```python
from build123d import *

# Parameters (mm, degrees)
BASE_DEPTH                = 12
CASE_MOUNTING_HOLES_REACH = 24.858
SKETCH2_R                 = 1.4
F_1MM_EDGE_FILLETS_R      = 1


with BuildPart() as part:
    # Sketch1 → Base (new body)
    with BuildSketch(Plane(origin=(0, 0, 0), x_dir=(1, 0, 0), z_dir=(0, 1, 0))):
        with BuildLine():
            Line((8.5, 17.5), (8.5, 15.5))
            ThreePointArc((8.5, 15.5), (7.297918472, 15.002081528), (6.8, 13.8))
            Line((6.8, 13.8), (6.8, 11.2))
            ThreePointArc((6.8, 11.2), (7.297918472, 9.997918472), (8.5, 9.5))
            Line((8.5, 9.5), (8.5, -9.5))
            ThreePointArc((8.5, -9.5), (7.297918472, -9.997918472), (6.8, -11.2))
            Line((6.8, -11.2), (6.8, -13.8))
            ThreePointArc((6.8, -13.8), (7.297918472, -15.002081528), (8.5, -15.5))
            Line((8.5, -15.5), (8.5, -17.5))
            Line((8.5, -17.5), (0, -17.5))
            Line((0, -17.5), (0, 17.5))
            Line((0, 17.5), (8.5, 17.5))
        make_face()
    extrude(amount=BASE_DEPTH)

    # Sketch2 → Case Mounting Holes (cut, up to next)
    with BuildSketch(Plane(origin=(8.5, 0, 0), x_dir=(0, 0, -1), z_dir=(1, 0, 0)), mode=Mode.PRIVATE) as case_mounting_holes_sk1:
        with Locations((-4.5, 6)):
            Circle(SKETCH2_R)
    case_mounting_holes_tool1 = extrude(case_mounting_holes_sk1.sketch, amount=-CASE_MOUNTING_HOLES_REACH, mode=Mode.PRIVATE) & part.part
    # Sketch2 → Case Mounting Holes (cut, up to next)
    with BuildSketch(Plane(origin=(8.5, 0, 0), x_dir=(0, 0, -1), z_dir=(1, 0, 0)), mode=Mode.PRIVATE) as case_mounting_holes_sk2:
        with Locations((4.5, 6)):
            Circle(SKETCH2_R)
    case_mounting_holes_tool2 = extrude(case_mounting_holes_sk2.sketch, amount=-CASE_MOUNTING_HOLES_REACH, mode=Mode.PRIVATE) & part.part
    add(case_mounting_holes_tool1.solids().sort_by_distance((8.5, 6, 4.5))[0], mode=Mode.SUBTRACT)
    add(case_mounting_holes_tool2.solids().sort_by_distance((8.5, 6, -4.5))[0], mode=Mode.SUBTRACT)

    # 1mm Edge Fillets
    f_1mm_edge_fillets_edges = [part.edges().sort_by_distance(p)[0] for p in [
        (4.25, 0, -17.5),
        (4.25, 0, 17.5),
        (4.25, 12, -17.5),
        (4.25, 12, 17.5),
    ]]
    fillet(f_1mm_edge_fillets_edges, radius=F_1MM_EDGE_FILLETS_R)


solid = part.part
```
Input: part model. Units: mm. Frame: model coordinates. A direction names the side the tool comes from. Give positions to 0.01 mm unless a question says otherwise; leave off trailing zeros. Loops run counter-clockwise (first coordinate to the right, second up) from the corner with the lowest first, then second, coordinate; pieces in that order, holes last.
1) Reachability of faces 1 (the flat face through (6.8, 6, -13)), 2 (the flat face through (8.5, 6, -17)) from +Z, -Z, +X, -X, +Y, -Y: full face, straight path, thin tool, end or side. Return the list, or none.
A:
face 1: +X, +Y, -Y
face 2: +Z, -Z, +X, +Y, -Y
2) Section query C-C on z = -4.5. Return the cut outline in (x, y), and give its area (3 significant figures).
A:
outline: (0, 0) - (8.5, 0) - (8.5, 4.6) - (0, 4.6) - close; (0, 7.4) - (8.5, 7.4) - (8.5, 12) - (0, 12) - close
area: 78.2 mm2
3) Line query: L1, parallel to Y at x = 6.75, z = -4.5; L2, parallel to Z at x = 1.75, y = 4.75; L3, parallel to Z at x = 7.5, y = 2.5. Output: solid intervals per line, ascending.
A:
L1: y = 0 to 4.6, 7.4 to 12
L2: z = -17.5 to -5.13, -3.87 to 3.87, 5.13 to 17.5
L3: z = -17.5 to -15.17, -9.83 to 9.83, 15.17 to 17.5
4) Mould query, pull axis Z, two halves, no side actions, for faces 3 (the cylindrical face through (4.19, 11.715, 17.199)), 4 (the flat face through (4, 6, -17.5)), 5 (the flat face through (6.8, 6, 12)). Classes: released by +Z, released by -Z, zero draft, split by the parting line, or undercut.
A:
face 3: released by +Z
face 4: released by -Z
face 5: undercut
5) Section query A-A on y = 6. Return the cut outline in (x, z).
A:
outline: (0, -17.5) - (8.5, -17.5) - (8.5, -15.5) arc R1.7 cw to (6.8, -13.8) - (6.8, -11.2) arc R1.7 cw to (8.5, -9.5) - (8.5, -5.9) - (0, -5.9) - close; (0, -3.1) - (8.5, -3.1) - (8.5, 3.1) - (0, 3.1) - close; (0, 5.9) - (8.5, 5.9) - (8.5, 9.5) arc R1.7 cw to (6.8, 11.2) - (6.8, 13.8) arc R1.7 cw to (8.5, 15.5) - (8.5, 17.5) - (0, 17.5) - close
6) Contact query for flat-ended pins moving along their axis: pin 1 (3.5 mm diameter, centred on y = 6, z = 4.5, fed in from +X); pin 2 (1.5 mm diameter, centred on y = 5.5, z = 11, fed in from +X); pin 3 (3 mm diameter, centred on y = 3, z = 12.5, fed in from +X). Output: stop coordinate, or through.
A:
pin 1: stops at x = 8.5
pin 2: stops at x = 7.09
pin 3: stops at x = 6.81
7) Section query B-B on x = 1.25. Return the cut outline in (y, z).
A:
outline: (0, -16.5) arc R1 ccw to (1, -17.5) - (11, -17.5) arc R1 ccw to (12, -16.5) - (12, 16.5) arc R1 ccw to (11, 17.5) - (1, 17.5) arc R1 ccw to (0, 16.5) - close; hole circle Ø2.8 at (6, -4.5); hole circle Ø2.8 at (6, 4.5)
8) Section query D-D on y = 8.75. Return the cut outline in (x, z), and give its area (3 significant figures).
A:
outline: (0, -17.5) - (8.5, -17.5) - (8.5, -15.5) arc R1.7 cw to (6.8, -13.8) - (6.8, -11.2) arc R1.7 cw to (8.5, -9.5) - (8.5, 9.5) arc R1.7 cw to (6.8, 11.2) - (6.8, 13.8) arc R1.7 cw to (8.5, 15.5) - (8.5, 17.5) - (0, 17.5) - close
area: 280 mm2
